Can you work these out from the model? Positions are in its coordinate system, mm. Coordinates: 2 decimals unless noted, no trailing zeros. Order: outer loops, then holes, each group sorted by start corner. A loop starts at its lowest first (then second) coordinate and runs counter-clockwise, first axis right, second up. Notation, with made-up numbers: (75, 34) -> (79, 34) arc R8 cw to (79, 47) -> close; hole circle Ø11 at (-20, 2.25). An arc over 180 degrees is marked (long way). Write item = value, one per line.
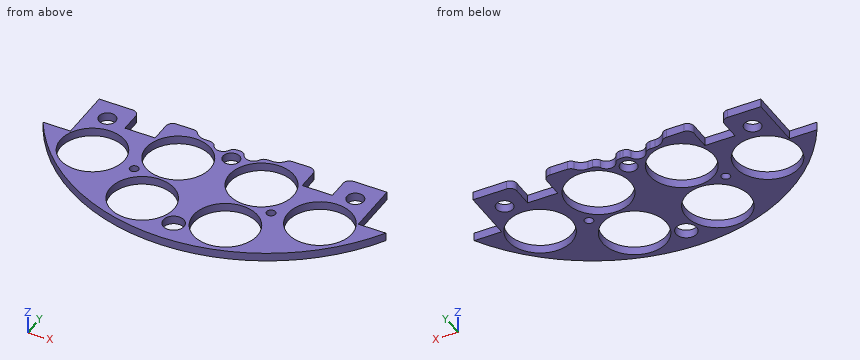
```python
from build123d import *

# Parameters (mm, degrees)
SKETCH1_R                = 1.651
BOSS_EXTRUDE2_DEPTH      = 3.175
SKETCH2_R                = 1.143
CUT_EXTRUDE1_DEPTH       = 4.175
SKETCH3_R                = 12.1285
CUT_EXTRUDE2_DEPTH       = 4.175
SKETCH4_W                = 28.562713242
SKETCH4_H                = 11.677503754
BOSS_EXTRUDE3_DEPTH      = 3.175
SKETCH5_W                = 216.7214489
SKETCH5_H                = 130.569220634
CUT_EXTRUDE4_DEPTH       = 4.175
SKETCH11_R               = 3.937
CUT_EXTRUDE11_DEPTH      = 4.175
SKETCH12_W               = 11.43
SKETCH12_H               = 10.16
CUT_EXTRUDE12_DEPTH      = 4.175
SKETCH16_R               = 12.192
CUT_EXTRUDE16_DEPTH      = 21.59
SKETCH57_R               = 1.651
CUT_EXTRUDE57_DEPTH      = 58.674
SKETCH58_R               = 3.175
CUT_EXTRUDE58_DEPTH      = 103.378
CUT_EXTRUDE58_DEPTH_BACK = 48.768
CUT_EXTRUDE15_DEPTH      = 21.59
FILLET1_R                = 2.54


with BuildPart() as part:
    # Sketch1 → Boss-Extrude2 (new body)
    with BuildSketch(Plane.XY):
        with BuildLine():
            Line((-64.964441474, 37.338), (-54.550441474, 37.338))
            Line((-54.550441474, 37.338), (-54.550441474, -37.338))
            Line((-54.550441474, -37.338), (-64.964441474, -37.338))
            ThreePointArc((-64.964441474, -37.338), (0, -74.93), (64.964441474, -37.338))
            Line((64.964441474, -37.338), (54.550441474, -37.338))
            Line((54.550441474, -37.338), (54.550441474, 37.338))
            Line((54.550441474, 37.338), (64.964441474, 37.338))
            ThreePointArc((64.964441474, 37.338), (0, 74.93), (-64.964441474, 37.338))
        make_face()
        with Locations((-46.482, 11.049)):
            Circle(SKETCH1_R, mode=Mode.SUBTRACT)
        with Locations((-21.083270032, 10.795)):
            Circle(SKETCH1_R, mode=Mode.SUBTRACT)
        with Locations((-21.083270032, -10.795)):
            Circle(SKETCH1_R, mode=Mode.SUBTRACT)
        with Locations((-46.482, -11.049)):
            Circle(SKETCH1_R, mode=Mode.SUBTRACT)
        with Locations((46.482, -11.049)):
            Circle(SKETCH1_R, mode=Mode.SUBTRACT)
        with Locations((21.083270032, -10.795)):
            Circle(SKETCH1_R, mode=Mode.SUBTRACT)
        with Locations((21.083270032, 10.795)):
            Circle(SKETCH1_R, mode=Mode.SUBTRACT)
        with Locations((46.482, 11.049)):
            Circle(SKETCH1_R, mode=Mode.SUBTRACT)
    extrude(amount=BOSS_EXTRUDE2_DEPTH)

    # Sketch2 → Cut-Extrude1 (cut, through all)
    with BuildSketch(Plane.XY.offset(3.175)):
        with Locations((-6.731, 62.23)):
            Circle(SKETCH2_R)
        with Locations((6.731, 62.23)):
            Circle(SKETCH2_R)
    extrude(amount=-CUT_EXTRUDE1_DEPTH, mode=Mode.SUBTRACT)

    # Sketch3 → Cut-Extrude2 (cut, through all)
    with BuildSketch(Plane(origin=(0, 0, 0), x_dir=(-1, 0, 0), z_dir=(0, 0, -1))):
        with Locations((-15.777608989, -58.882838371)):
            Circle(SKETCH3_R)
        with Locations((15.777608989, -58.882838371)):
            Circle(SKETCH3_R)
        with Locations((-43.105229381, -43.105229381)):
            Circle(SKETCH3_R)
        with Locations((-43.105229381, 43.105229381)):
            Circle(SKETCH3_R)
        with Locations((43.105229381, 43.105229381)):
            Circle(SKETCH3_R)
        with Locations((43.105229381, -43.105229381)):
            Circle(SKETCH3_R)
    extrude(amount=-CUT_EXTRUDE2_DEPTH, mode=Mode.SUBTRACT)

    # Sketch4 → Boss-Extrude3 (add)
    with BuildSketch(Plane(origin=(0, 0, 0), x_dir=(-1, 0, 0), z_dir=(0, 0, -1))):
        with Locations((-1.488809975, 62.152540216)):
            Rectangle(SKETCH4_W, SKETCH4_H)
    extrude(amount=-BOSS_EXTRUDE3_DEPTH)

    # Sketch5 → Cut-Extrude4 (cut, through all)
    with BuildSketch(Plane(origin=(0, 0, 0), x_dir=(-1, 0, 0), z_dir=(0, 0, -1))):
        with Locations((23.316688373, 48.139610317)):
            Rectangle(SKETCH5_W, SKETCH5_H)
    extrude(amount=-CUT_EXTRUDE4_DEPTH, mode=Mode.SUBTRACT)

    # Sketch11 → Cut-Extrude11 (cut, through all)
    with BuildSketch(Plane(origin=(0, 0, 0), x_dir=(-1, 0, 0), z_dir=(0, 0, -1))):
        with Locations((0, -66.045)):
            Circle(SKETCH11_R)
    extrude(amount=-CUT_EXTRUDE11_DEPTH, mode=Mode.SUBTRACT)

    # Sketch12 → Cut-Extrude12 (cut, through all)
    with BuildSketch(Plane(origin=(0, 0, 0), x_dir=(-1, 0, 0), z_dir=(0, 0, -1))):
        with Locations((-33.595441474, -22.225)):
            Rectangle(SKETCH12_W, SKETCH12_H)
        with Locations((33.595441474, -22.225)):
            Rectangle(SKETCH12_W, SKETCH12_H)
    extrude(amount=-CUT_EXTRUDE12_DEPTH, mode=Mode.SUBTRACT)

    # Sketch16 → Cut-Extrude16 (cut)
    with BuildSketch(Plane(origin=(0, 0, 0), x_dir=(-1, 0, 0), z_dir=(0, 0, -1))):
        with Locations((15.777608989, -33.482838371)):
            Circle(SKETCH16_R)
        with Locations((-15.777608989, -33.482838371)):
            Circle(SKETCH16_R)
    extrude(amount=-CUT_EXTRUDE16_DEPTH, mode=Mode.SUBTRACT)

    # Sketch57 → Cut-Extrude57 (cut)
    with BuildSketch(Plane(origin=(0, 0, 0), x_dir=(-1, 0, 0), z_dir=(0, 0, -1))):
        with Locations((-25.937608989, -45.645229381)):
            Circle(SKETCH57_R)
        with Locations((25.937608989, -45.645229381)):
            Circle(SKETCH57_R)
    extrude(amount=-CUT_EXTRUDE57_DEPTH, mode=Mode.SUBTRACT)

    # Sketch58 → Cut-Extrude58 (cut, two sides)
    with BuildSketch(Plane(origin=(30.092005081, 4.08352975, 36.1315), x_dir=(-1, 0, 0), z_dir=(0, 0, -1))) as cut_extrude58_sk:
        with Locations((77.082005081, -29.48352975)):
            Circle(SKETCH58_R)
        with Locations((30.092005081, -29.48352975)):
            Circle(SKETCH58_R)
        with Locations((-16.897994919, -29.48352975)):
            Circle(SKETCH58_R)
    extrude(amount=CUT_EXTRUDE58_DEPTH, mode=Mode.SUBTRACT)
    extrude(cut_extrude58_sk.sketch, amount=-CUT_EXTRUDE58_DEPTH_BACK, mode=Mode.SUBTRACT)

    # Sketch15 → Cut-Extrude15 (cut)
    with BuildSketch(Plane(origin=(0, 0, 0), x_dir=(-1, 0, 0), z_dir=(0, 0, -1))):
        with BuildLine():
            Line((-12.7, -20.24), (-8.888991966, -20.24))
            ThreePointArc((-8.888991966, -20.24), (-5.715, -23.495), (-2.541008034, -20.24))
            Line((-2.541008034, -20.24), (2.541008034, -20.24))
            ThreePointArc((2.541008034, -20.24), (5.715, -23.495), (8.888991966, -20.24))
            Line((8.888991966, -20.24), (12.7, -20.24))
            ThreePointArc((12.7, -20.24), (16.235533906, -11.704466094), (7.7, -15.24))
            Line((7.7, -15.24), (-1.06, -15.24))
            ThreePointArc((-1.06, -15.24), (-4.010609847, -10.6792983), (-9.38, -11.501337137))
            ThreePointArc((-9.38, -11.501337137), (-17.374040774, -13.464234575), (-12.7, -20.24))
        make_face()
    extrude(amount=-CUT_EXTRUDE15_DEPTH, mode=Mode.SUBTRACT)

    # Fillet1
    fillet1_edges = [part.edges().sort_by_distance(p)[0] for p in [
        (39.310441474, -17.145, 1.5875),
        (27.880441474, -17.145, 1.5875),
        (-27.880441474, -17.145, 1.5875),
        (-39.310441474, -17.145, 1.5875),
        (-17.322875188, -17.145, 1.5875),
        (17.322875188, -17.145, 1.5875),
        (-8.888991966, -20.24, 1.5875),
        (-2.541008034, -20.24, 1.5875),
        (2.541008034, -20.24, 1.5875),
        (8.888991966, -20.24, 1.5875),
    ]]
    fillet(fillet1_edges, radius=FILLET1_R)


solid = part.part
```
Item 1: If I drill on probe 1 along Y at (x, z) = (10, 0.5); probe 2 along X at (y, z) = (-56, 2.75); probe 3 along X at (y, z) = (-68, 1.55), over which ranges is the centre line in solid material (lowest first)?
A:
probe_1 = -74.26 to -69.55, -48.22 to -44.22, -22.75 to -20.39
probe_2 = -49.78 to -27.56, -4 to 4, 27.56 to 49.78
probe_3 = -31.47 to -23.78, -7.78 to -3.42, 3.42 to 7.78, 23.78 to 31.47
Item 2: I want a section at D-D, the plane x = -21.5. Please give me the cut outline in (y, z) (3 decimals).
A:
outline = (-71.779, 0) -> (-69.577, 0) -> (-69.577, 3.175) -> (-71.779, 3.175) -> close; (-48.189, 0) -> (-44.248, 0) -> (-44.248, 3.175) -> (-48.189, 3.175) -> close; (-22.717, 0) -> (-17.145, 0) -> (-17.145, 3.175) -> (-22.717, 3.175) -> close
Item 3: I want a section at B-B, the plane x = 48.5. Please give me the cut outline in (y, z) (3 decimals).
A:
outline = (-57.116, 0) -> (-53.968, 0) -> (-53.968, 3.175) -> (-57.116, 3.175) -> close; (-32.243, 0) -> (-28.193, 0) -> (-28.193, 3.175) -> (-32.243, 3.175) -> close; (-22.607, 0) -> (-17.145, 0) -> (-17.145, 3.175) -> (-22.607, 3.175) -> close
Item 4: I want a section at A-A, the plane y = -35. Please give me the cut outline in (x, z) (3 decimals).
A:
outline = (-54.55, 0) -> (-52.128, 0) -> (-52.128, 3.175) -> (-54.55, 3.175) -> close; (-34.083, 0) -> (-27.875, 0) -> (-27.875, 3.175) -> (-34.083, 3.175) -> close; (-3.68, 0) -> (3.68, 0) -> (3.68, 3.175) -> (-3.68, 3.175) -> close; (27.875, 0) -> (34.083, 0) -> (34.083, 3.175) -> (27.875, 3.175) -> close; (52.128, 0) -> (54.55, 0) -> (54.55, 3.175) -> (52.128, 3.175) -> close
Item 5: I want a section at C-C, the plane y = -25.4. Give the number of separate pieces and of enclosed holes in the cut face, plus the area to 3 significant figures.
A:
separate_pieces = 8
enclosed_holes = 0
area = 97.4 mm2
Item 6: I'm going to push flat-ended pins straight in: P1, Ø19.5, axis at x = -15.78, y = -58.88, coming from the -Z side; P2, Ø0.9, axis at x = 12, z = 1.5, coming from the +Y side; P3, Ø1, axis at y = -55.5, z = 2.5, coming from the +X side; P4, Ø1, axis at y = -21.5, z = 1.5, coming from the -X side. Where does each tip first touch, or does it pass through?
A:
P1 = through
P2 = -20.24
P3 = 50.89
P4 = -54.55
